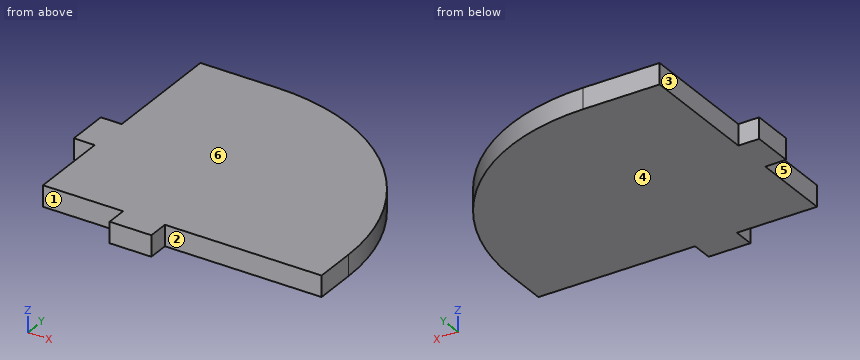
from build123d import *

# Parameters (mm, degrees)
EXTRUDE_1_DEPTH = 3


with BuildPart() as part:
    # 草图1 → 凸台-拉伸1 (new body)
    with BuildSketch(Plane.XY):
        with BuildLine():
            Line((0, 17.5), (-3, 17.5))
            Line((-3, 17.5), (-3, 11.5))
            Line((-3, 11.5), (0, 11.5))
            Line((0, 11.5), (0, 0))
            Line((0, 0), (11.5, 0))
            Line((11.5, 0), (11.5, -3))
            Line((11.5, -3), (17.5, -3))
            Line((17.5, -3), (17.5, 0))
            Line((17.5, 0), (40, 0))
            Line((40, 0), (40, 6))
            ThreePointArc((40, 6), (31.506096654, 26.506096654), (11, 35))
            Line((11, 35), (0, 35))
            Line((0, 35), (0, 17.5))
        make_face()
    extrude(amount=EXTRUDE_1_DEPTH)


solid = part.part
CAD build for the part. Positions are in the model's coordinates, mm. Face numbers are marked on the shaded views. A direction names the side the tool comes from. Coordinates: 2 decimals unless noted, no trailing zeros. Write each loop counter-clockwise with the first axis right and the second up, starting at its lowest first coordinate (ties: lowest second). Pieces come first, ordered by that corner, then holes. Notation, with made-up numbers: (-20, -4.5) - (38, -4.5) arc R34 ccw to (38, 33.5) - close; hole circle Ø8 at (56, -35). An arc over 180 degrees is marked (long way). Use a Markdown table: item, result. Add a question column.
Item 1: Flat gauge pins, fed straight in: pin 1 (0.9 mm diameter, centred on y = -1.5, z = 1, fed in from -X); pin 2 (1 mm diameter, centred on y = 11, z = 0.5, fed in from +X); pin 3 (1.5 mm diameter, centred on x = -1.5, z = 2, fed in from -Y). Where does each tip first touch, or does it go through?
Item 2: Band-saw the part on A-A, the plane z = 2.05. Give the cut face in (x, y).
Item 3: Band-saw the part on C-C, the plane y = 27. Give the cut face in (x, z), and give its area (3 significant figures).
Item 4: Drill centre lines: L1, parallel to X at y = 4, z = 0.5; L2, parallel to Y at x = 1, z = 0.3; L3, parallel to X at y = 17, z = 2.2. Where is each one in solid material? Low to high. Write a range as from..to.
Item 5: 3-axis set-ups, long thin cutter, end or side, ignore diameter. For the marked faces 1, 2 and 3: which of +Z, -Z, +X, -X, +Y, -Y reach the whole face in a straight line?
Item 6: Mould opens along Z. For the marked faces 4, 5 and 6 say: pulls with the +Z half, pulls with the -Z half, needs draft (parallel to the pull), parting line crosses it, or undercut.
Item 7: Band-saw the part on B-B, the plane x = 6. Give the cut face in (y, z).
Numbers:
| question | item | result |
|---|---|---|
| 1 | pin 1 | x = 11.5 |
| 1 | pin 2 | x = 39.65 |
| 1 | pin 3 | y = 11.5 |
| 2 | outline | (-3, 11.5) - (0, 11.5) - (0, 0) - (11.5, 0) - (11.5, -3) - (17.5, -3) - (17.5, 0) - (40, 0) - (40, 6) arc R29 ccw to (11, 35) - (0, 35) - (0, 17.5) - (-3, 17.5) - close |
| 3 | outline | (0, 0) - (31, 0) - (31, 3) - (0, 3) - close |
| 3 | area | 93.0 mm2 |
| 4 | L1 | 0..40 |
| 4 | L2 | 0..35 |
| 4 | L3 | -3..37.83 |
| 5 | face 1 | +Z, -Z, -X, -Y |
| 5 | face 2 | +Z, -Z, +X, -Y |
| 5 | face 3 | +Z, -Z, -X, +Y |
| 6 | face 4 | pulls with the -Z half |
| 6 | face 5 | needs draft |
| 6 | face 6 | pulls with the +Z half |
| 7 | outline | (0, 0) - (35, 0) - (35, 3) - (0, 3) - close |
